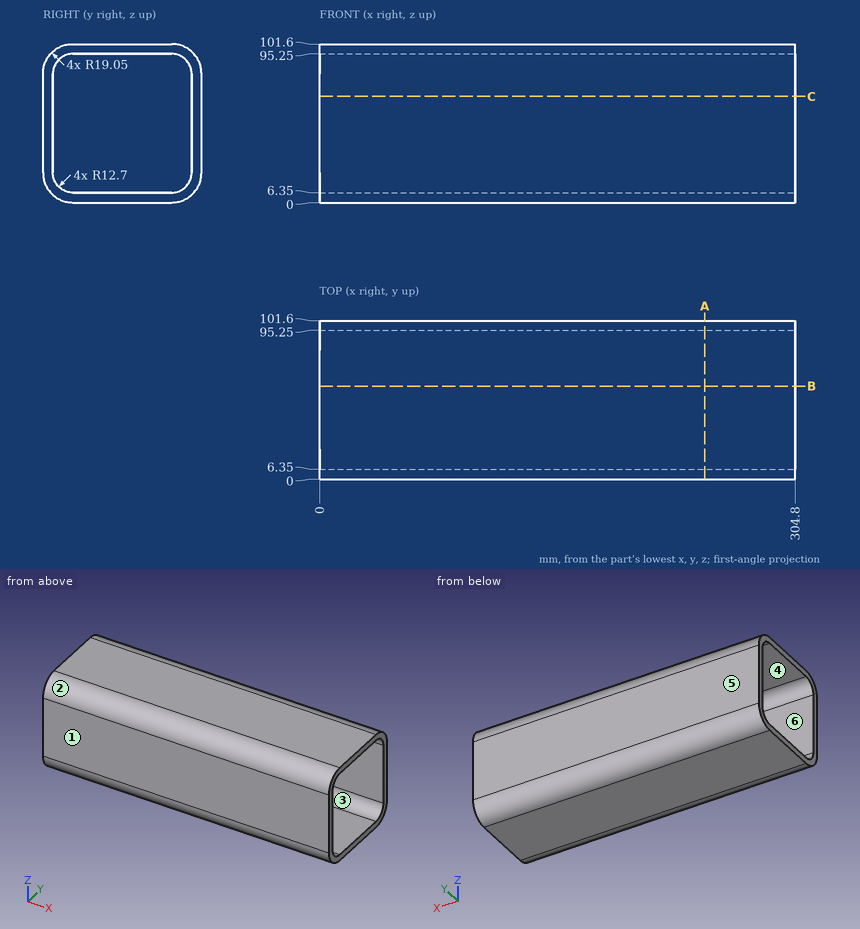
Could you check a few things on this drawing? It's one solid part, dimensions in mm from its lowest x, y, z. A direction names the side the tool comes from. Coordinates: 2 decimals unless noted, no trailing zeros. Order: outer loops, then holes, each group sorted by start corner. A loop starts at its lowest first (then second) coordinate and runs counter-clockwise, first axis right, second up. Notation, with made-up numbers: M 47,1.5 L 100,1.5 A23 ccw 100,19.5 Z; hole C -5.75,60 d11. An arc over 180 degrees is marked long. Use a Markdown table: item, result. Add a question column.
Q1. I want a section at A-A on x = 247. List the corners of the cut face in (y, z) for me, then the cut area to 3 significant figures.
Q2. We'd pull the mould along Z, two halves only. Please class the marked faces 1, 2, 3 and 4: pulls with the +Z half, pulls with the -Z half, needs draft (parallel to the pull), parting line crosses it, or undercut.
Q3. I want a section at B-B on y = 59.5. List the corners of the cut face in (x, z) for me.
Q4. Which directions (+Z, -Z, +X, -X, +Y, -Y) give clear straight access to the entire face, cutting with the end or side of a thin tool? Please do the marked faces 5 and 6.
Q5. I'm going to push a flat-ended pin straight in: pin 1 (2 mm diameter, centred on x = 94, z = 88.5, fed in from +Y). Where does the tip first touch, or does it pass through?
Q6. If I drill on L1, parallel to Z at x = 30.5, y = 48.5; L2, parallel to Y at x = 168, z = 6, over which ranges is the centre line in solid material (lowest first)?
Checked values:
| question | item | result |
|---|---|---|
| 1 | outline | M 0,19.05 A19.05 ccw 19.05,0 L 82.55,0 A19.05 ccw 101.6,19.05 L 101.6,82.55 A19.05 ccw 82.55,101.6 L 19.05,101.6 A19.05 ccw 0,82.55 Z; hole M 6.35,19.05 A12.7 ccw 19.05,6.35 L 82.55,6.35 A12.7 ccw 95.25,19.05 L 95.25,82.55 A12.7 ccw 82.55,95.25 L 19.05,95.25 A12.7 ccw 6.35,82.55 Z |
| 1 | area | 2,250 mm² |
| 2 | face 1 | needs draft |
| 2 | face 2 | pulls with the +Z half |
| 2 | face 3 | undercut |
| 2 | face 4 | undercut |
| 3 | outline | M 0,0 L 304.8,0 L 304.8,6.35 L 0,6.35 Z; M 0,95.25 L 304.8,95.25 L 304.8,101.6 L 0,101.6 Z |
| 4 | face 5 | +Z, -Z, +X, -X, +Y |
| 4 | face 6 | +X, -X |
| 5 | pin 1 | y = 100.95 |
| 6 | L1 | 0 to 6.35, 95.25 to 101.6 |
| 6 | L2 | 5.17 to 96.43 |
